from build123d import *

# Parameters (mm, degrees)
SKIZZE1_R                         = 3
AUFSATZ_LINEAR_AUSTRAGEN1_DEPTH   = 5
AUFSATZ_LINEAR_AUSTRAGEN1_2_DEPTH = 5
AUFSATZ_LINEAR_AUSTRAGEN1_3_DEPTH = 5
SKIZZE2_W                         = 6
SKIZZE2_H                         = 12.7
AUFSATZ_LINEAR_AUSTRAGEN2_DEPTH   = 4
SKIZZE3_W                         = 20.32
SKIZZE3_H                         = 6
AUFSATZ_LINEAR_AUSTRAGEN3_DEPTH   = 4
AUFSATZ_LINEAR_AUSTRAGEN6_DEPTH   = 4
SKIZZE10_R                        = 3
AUFSATZ_LINEAR_AUSTRAGEN7_DEPTH   = 4
SKIZZE11_R                        = 1.7
SCHNITT_LINEAR_AUSTRAGEN5_DEPTH   = 4
SKIZZE12_R                        = 1.15
SCHNITT_LINEAR_AUSTRAGEN6_DEPTH   = 5
SKIZZE14_R                        = 1.15
SCHNITT_LINEAR_AUSTRAGEN8_DEPTH   = 6
SKIZZE15_R                        = 3
SKIZZE15_R_2                      = 1.15
AUFSATZ_LINEAR_AUSTRAGEN9_DEPTH   = 8.13
SKIZZE19_W                        = 52.396987113
SKIZZE19_H                        = 51.888823268
SCHNITT_LINEAR_AUSTRAGEN12_DEPTH  = 4.13


with BuildPart() as part:
    # Skizze1 → Aufsatz-Linear austragen1 (new body)
    with BuildSketch(Plane.XY):
        with Locations((-2.54, 2.54)):
            Circle(SKIZZE1_R)
    extrude(amount=AUFSATZ_LINEAR_AUSTRAGEN1_DEPTH)



with BuildPart() as body_2:
    # Skizze1 → Aufsatz-Linear austragen1 2 (new body)
    with BuildSketch(Plane.XY):
        with Locations((-2.54, 15.24)):
            Circle(SKIZZE1_R)
    extrude(amount=AUFSATZ_LINEAR_AUSTRAGEN1_2_DEPTH)


with BuildPart() as body_3:
    # Skizze1 → Aufsatz-Linear austragen1 3 (new body)
    with BuildSketch(Plane.XY):
        with Locations((-22.86, 2.54)):
            Circle(SKIZZE1_R)
    extrude(amount=AUFSATZ_LINEAR_AUSTRAGEN1_3_DEPTH)


with BuildPart() as part_1:
    add(part.part)

    add(body_2.part)  # Aufsatz-Linear austragen2 merges body 2
    # Skizze2 → Aufsatz-Linear austragen2 (add)
    with BuildSketch(Plane.XY.offset(5)):
        with Locations((-2.54, 8.89)):
            Rectangle(SKIZZE2_W, SKIZZE2_H)
    extrude(amount=-AUFSATZ_LINEAR_AUSTRAGEN2_DEPTH)

    # Skizze3 → Aufsatz-Linear austragen3 (add)
    with BuildSketch(Plane.XY.offset(5)):
        with Locations((-12.7, 2.54)):
            Rectangle(SKIZZE3_W, SKIZZE3_H)
    extrude(amount=-AUFSATZ_LINEAR_AUSTRAGEN3_DEPTH)


    add(body_3.part)  # Aufsatz-Linear austragen6 merges body 3
    # Skizze9 → Aufsatz-Linear austragen6 (add)
    with BuildSketch(Plane(origin=(0, 0, 1), x_dir=(-1, 0, 0), z_dir=(0, 0, -1))):
        with BuildLine():
            Line((21.403833859, -0.082895379), (24.316166141, 5.162895379))
            ThreePointArc((24.316166141, 5.162895379), (34.161496772, -4.480544132), (37.695021225, -17.801229766))
            ThreePointArc((37.695021225, -17.801229766), (34.668329668, -20.774298587), (31.695260847, -17.747607029))
            ThreePointArc((31.695260847, -17.747607029), (28.977165113, -7.500925772), (21.403833859, -0.082895379))
        make_face()
    extrude(amount=-AUFSATZ_LINEAR_AUSTRAGEN6_DEPTH)

    # Skizze10 → Aufsatz-Linear austragen7 (add)
    with BuildSketch(Plane(origin=(0, 0, 1), x_dir=(-1, 0, 0), z_dir=(0, 0, -1))):
        with Locations((34.695141036, -17.774418398)):
            Circle(SKIZZE10_R)
    extrude(amount=-AUFSATZ_LINEAR_AUSTRAGEN7_DEPTH)

    # Skizze11 → Schnitt-Linear austragen5 (cut)
    with BuildSketch(Plane(origin=(0, 0, 0), x_dir=(-1, 0, 0), z_dir=(0, 0, -1))):
        with Locations((2.54, 15.24)):
            Circle(SKIZZE11_R)
        with Locations((22.86, 2.54)):
            Circle(SKIZZE11_R)
    extrude(amount=-SCHNITT_LINEAR_AUSTRAGEN5_DEPTH, mode=Mode.SUBTRACT)

    # Skizze12 → Schnitt-Linear austragen6 (cut, through all)
    with BuildSketch(Plane(origin=(0, 0, 1), x_dir=(-1, 0, 0), z_dir=(0, 0, -1))):
        with Locations((34.695141036, -17.774418398)):
            Circle(SKIZZE12_R)
    extrude(amount=-SCHNITT_LINEAR_AUSTRAGEN6_DEPTH, mode=Mode.SUBTRACT)

    # Skizze14 → Schnitt-Linear austragen8 (cut, through all)
    with BuildSketch(Plane(origin=(0, 0, 0), x_dir=(-1, 0, 0), z_dir=(0, 0, -1))):
        with Locations((2.54, 2.54)):
            Circle(SKIZZE14_R)
    extrude(amount=-SCHNITT_LINEAR_AUSTRAGEN8_DEPTH, mode=Mode.SUBTRACT)

    # Skizze15 → Aufsatz-Linear austragen9 (add)
    with BuildSketch(Plane(origin=(0, 0, 0), x_dir=(-1, 0, 0), z_dir=(0, 0, -1))):
        with Locations((2.54, 2.54)):
            Circle(SKIZZE15_R)
        with Locations((2.54, 2.54)):
            Circle(SKIZZE15_R_2, mode=Mode.SUBTRACT)
    extrude(amount=-AUFSATZ_LINEAR_AUSTRAGEN9_DEPTH)

    # Skizze19 → Schnitt-Linear austragen12 (cut, through all)
    with BuildSketch(Plane.XY.offset(5)):
        with Locations((-20.173492866, -0.896131467)):
            Rectangle(SKIZZE19_W, SKIZZE19_H)
    extrude(amount=SCHNITT_LINEAR_AUSTRAGEN12_DEPTH, mode=Mode.SUBTRACT)


solid = part_1.part
Source: CAD feature listing. Evaluate the final solid. Frame: model axes, mm. A direction names the side the tool comes from. Give positions to 0.01 mm unless a question says otherwise; leave off trailing zeros. Write each loop counter-clockwise with the first axis right and the second up, starting at its lowest first coordinate (ties: lowest second). Pieces come first, ordered by that corner, then holes. Notation, with made-up numbers: M 71.25,-11.5 L 108.25,-11.5 A16 cw 108.25,12.5 Z; hole C 53,2 d7. An arc over 180 degrees is marked long. Return JSON: item names as keys, results as strings. Group by question number.
1) Cut plane B-B, the plane y = 8. Output: boundary loops of the cut face in (x, z), then the cut area to 3 significant figures.
2) Set-up query: faces 1 (the face through (-35.792, -17.429, 2.972)), 2 (the face through (-19, 2, 5)), 3 (the face through (-5.54, 10, 3)), 4 (the face through (-12, -0.46, 3)), 5 (the face through (-2.931, 18.214, 1.909)). Return all of +Z, -Z, +X, -X, +Y, -Y with unobstructed straight access to the full face (end or side cutting, diameter ignored); none if empty.
3) First-contact query: pin 1 Ø1 at (y, z) = (9, 4) entering from -X; pin 2 Ø1 at (x, z) = (-27.5, 1) entering from +Y; pin 3 Ø3 at (x, z) = (-9, 3) entering from -Y. Flat tips, straight axial feed; report the tip coordinate or a pass-through.
4) Cut plane C-C, the plane x = -15.5. Output: boundary loops of the cut face in (y, z), then the cut area to 3 significant figures.
5) Cut plane A-A, the plane z = 0.5. Output: boundary loops of the cut face in (x, y).
6) Ray query, L1, parallel to X at y = 2, z = 4.1; L2, parallel to X at y = 4, z = 3.55; L3, parallel to Y at x = -22, z = 2.1. Return the intervals inside material, ascending.
Data:
{
 "1": {"outline": "M -5.54,1 L 0.46,1 L 0.46,5 L -5.54,5 Z", "area": "24.0 mm²"},
 "2": {"face 1": "+Z, -Z", "face 2": "+Z, +X, -X, +Y, -Y", "face 3": "+Z, -Z, -X, +Y", "face 4": "+Z, -Z, +X, -Y", "face 5": "-Z"},
 "3": {"pin 1": "stops at x = -5.54", "pin 2": "stops at y = 3.45", "pin 3": "stops at y = -0.46"},
 "4": {"outline": "M -0.46,1 L 5.54,1 L 5.54,5 L -0.46,5 Z", "area": "24.0 mm²"},
 "5": {"outline": "C -22.86,2.54 d6; C -2.54,2.54 d6; C -2.54,15.24 d6; hole C -22.86,2.54 d3.4; hole C -2.54,15.24 d3.4; hole C -2.54,2.54 d2.3"},
 "6": {"L1": "x = -28.82 to -3.56, -1.52 to 0.41", "L2": "x = -26.21 to -23.73, -21.99 to 0.46", "L3": "y = -0.46 to 1.07, 4.01 to 5.54"}
}
